Geometry check sheet. Reference: the model listing, model coordinates, mm. Face numbers are marked on the shaded views. A direction names the side the tool comes from. Round coordinates to 2 decimals unless told otherwise and drop trailing zeros. Write each loop counter-clockwise with the first axis right and the second up, starting at its lowest first coordinate (ties: lowest second). Pieces come first, ordered by that corner, then holes. Notation, with made-up numbers: M -3.75,12.25 L 19.25,12.25 A11 cw 19.25,20.25 Z; hole C 42.5,-12 d10. An arc over 180 degrees is marked long. One line per item, written item: value. Start each with the question number.
1. Scan lines: probe 1 along X at (y, z) = (11, 0.55); probe 2 along Y at (x, z) = (3, -0.3); probe 3 along Z at (x, y) = (1.5, 4.75). Record each from-to range of solid material in increasing order. Write a range as [from, to].
2. Section check A-A (x = 1). Record the boundary of the cut face in (y, z), and give its area (3 significant figures).
3. Section check D-D (x = 2.25). Record the boundary of the cut face in (y, z).
4. Depth check by flat-ended pin: P1, Ø0.8, axis at y = 8, z = 0.5, coming from the -X side; P2, Ø4, axis at x = -1, y = 9, coming from the +Z side; P3, Ø1.3, axis at y = 12.5, z = 0.5, coming from the -X side. Enter the tip coordinate at first touch or a pass-through.
5. Access from +Z, -Z, +X, -X, +Y, -Y to the whole of each face (thin tool, end or side, straight path). Record for the marked faces 1, 2, 3 and 4.
6. Section check B-B (z = -0.5). Record the boundary of the cut face in (x, y), and give its area (3 significant figures).
7. Section check C-C (y = 7). Record the boundary of the cut face in (x, z).
from build123d import *

# Parameters (mm, degrees)
SKETCH1_W           = 7.7
SKETCH1_H           = 2.5
BOSS_EXTRUDE1_DEPTH = 4.7
SKETCH2_W           = 4.8
SKETCH2_H           = 1.6
BOSS_EXTRUDE2_DEPTH = 4.5
SKETCH3_W           = 3.8
SKETCH3_H           = 1.6
BOSS_EXTRUDE3_DEPTH = 4.6


with BuildPart() as part:
    # Sketch1 → Boss-Extrude1 (new body)
    with BuildSketch(Plane(origin=(0, 0, 0), x_dir=(1, 0, 0), z_dir=(0, 1, 0))):
        Rectangle(SKETCH1_W, SKETCH1_H)
    extrude(amount=BOSS_EXTRUDE1_DEPTH)

    # Sketch2 → Boss-Extrude2 (add)
    with BuildSketch(Plane(origin=(0, 4.7, 0), x_dir=(1, 0, 0), z_dir=(0, 1, 0))):
        Rectangle(SKETCH2_W, SKETCH2_H)
    extrude(amount=BOSS_EXTRUDE2_DEPTH)

    # Sketch3 → Boss-Extrude3 (add)
    with BuildSketch(Plane(origin=(0, 9.2, 0), x_dir=(1, 0, 0), z_dir=(0, 1, 0))):
        Rectangle(SKETCH3_W, SKETCH3_H)
    extrude(amount=BOSS_EXTRUDE3_DEPTH)


solid = part.part
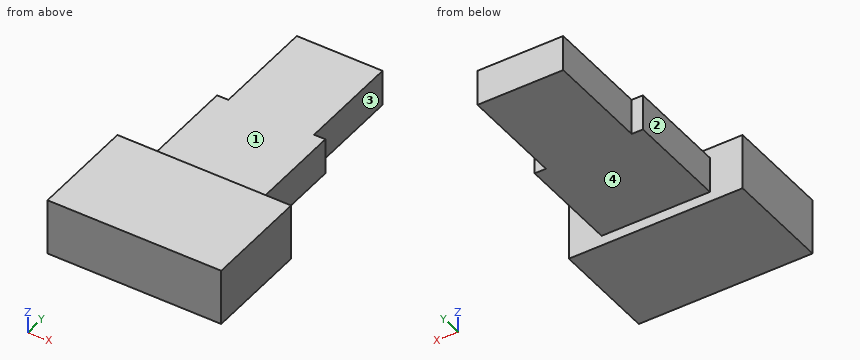
Result sheet:
1. probe 1: x = [-1.9, 1.9]
1. probe 2: y = [0, 4.7]
1. probe 3: z = [-0.8, 0.8]
2. outline: M 0,-1.25 L 4.7,-1.25 L 4.7,-0.8 L 13.8,-0.8 L 13.8,0.8 L 4.7,0.8 L 4.7,1.25 L 0,1.25 Z
2. area: 26.3 mm2
3. outline: M 0,-1.25 L 4.7,-1.25 L 4.7,-0.8 L 9.2,-0.8 L 9.2,0.8 L 4.7,0.8 L 4.7,1.25 L 0,1.25 Z
4. P1: stops at x = -2.4
4. P2: stops at z = 0.8
4. P3: stops at x = -1.9
5. face 1: +Z, +X, -X, +Y
5. face 2: +Z, -Z, -X, +Y
5. face 3: +Z, -Z, +X, +Y
5. face 4: -Z, +X, -X, +Y
6. outline: M -3.85,0 L 3.85,0 L 3.85,4.7 L 2.4,4.7 L 2.4,9.2 L 1.9,9.2 L 1.9,13.8 L -1.9,13.8 L -1.9,9.2 L -2.4,9.2 L -2.4,4.7 L -3.85,4.7 Z
6. area: 75.3 mm2
7. outline: M -2.4,-0.8 L 2.4,-0.8 L 2.4,0.8 L -2.4,0.8 Z
